from build123d import *

# Parameters (mm, degrees)
SKETCH1_W           = 56.4
SKETCH1_H           = 56.4
BOSS_EXTRUDE1_DEPTH = 56
SKETCH2_R           = 2.55
CUT_EXTRUDE1_DEPTH  = 6
SKETCH3_R           = 19.05
BOSS_EXTRUDE2_DEPTH = 1.6
SKETCH4_R           = 4
BOSS_EXTRUDE3_DEPTH = 23.9
FILLET1_R           = 4
SKETCH5_W           = 9.15
SKETCH5_H           = 9.15
CUT_EXTRUDE2_DEPTH  = 51
FILLET3_R           = 4
FILLET4_R           = 2


with BuildPart() as part:
    # Sketch1 → Boss-Extrude1 (new body)
    with BuildSketch(Plane.XY):
        Rectangle(SKETCH1_W, SKETCH1_H)
    extrude(amount=-BOSS_EXTRUDE1_DEPTH)

    # Sketch2 → Cut-Extrude1 (cut)
    with BuildSketch(Plane.XY):
        with Locations((-23.57, 23.57)):
            Circle(SKETCH2_R)
        with Locations((23.57, 23.57)):
            Circle(SKETCH2_R)
        with Locations((23.57, -23.57)):
            Circle(SKETCH2_R)
        with Locations((-23.57, -23.57)):
            Circle(SKETCH2_R)
    extrude(amount=-CUT_EXTRUDE1_DEPTH, mode=Mode.SUBTRACT)

    # Sketch3 → Boss-Extrude2 (add)
    with BuildSketch(Plane.XY):
        Circle(SKETCH3_R)
    extrude(amount=BOSS_EXTRUDE2_DEPTH)

    # Sketch4 → Boss-Extrude3 (add)
    with BuildSketch(Plane.XY.offset(1.6)):
        Circle(SKETCH4_R)
    extrude(amount=BOSS_EXTRUDE3_DEPTH)

    # Fillet1
    fillet1_edges = [part.edges().sort_by_distance(p)[0] for p in [
        (28.2, -28.2, -28),
        (-28.2, -28.2, -28),
        (-28.2, 28.2, -28),
        (28.2, 28.2, -28),
    ]]
    fillet(fillet1_edges, radius=FILLET1_R)

    # Sketch5 → Cut-Extrude2 (cut)
    with BuildSketch(Plane(origin=(0, 0, -56), x_dir=(-1, 0, 0), z_dir=(0, 0, -1))):
        with Locations((-23.625, 23.625)):
            Rectangle(SKETCH5_W, SKETCH5_H)
        with Locations((23.625, 23.625)):
            Rectangle(SKETCH5_W, SKETCH5_H)
        with Locations((23.625, -23.625)):
            Rectangle(SKETCH5_W, SKETCH5_H)
        with Locations((-23.625, -23.625)):
            Rectangle(SKETCH5_W, SKETCH5_H)
    extrude(amount=-CUT_EXTRUDE2_DEPTH, mode=Mode.SUBTRACT)

    # Fillet3
    fillet3_edges = [part.edges().sort_by_distance(p)[0] for p in [
        (-19.05, 19.05, -30.5),
        (19.05, 19.05, -30.5),
        (19.05, -19.05, -30.5),
        (-19.05, -19.05, -30.5),
    ]]
    fillet(fillet3_edges, radius=FILLET3_R)

    # Fillet4
    fillet4_edges = [part.edges().sort_by_distance(p)[0] for p in [
        (-28.2, 19.05, -30.5),
        (-19.05, 28.2, -30.5),
        (28.2, 19.05, -30.5),
        (19.05, 28.2, -30.5),
        (28.2, -19.05, -30.5),
        (19.05, -28.2, -30.5),
        (-28.2, -19.05, -30.5),
        (-19.05, -28.2, -30.5),
    ]]
    fillet(fillet4_edges, radius=FILLET4_R)


solid = part.part
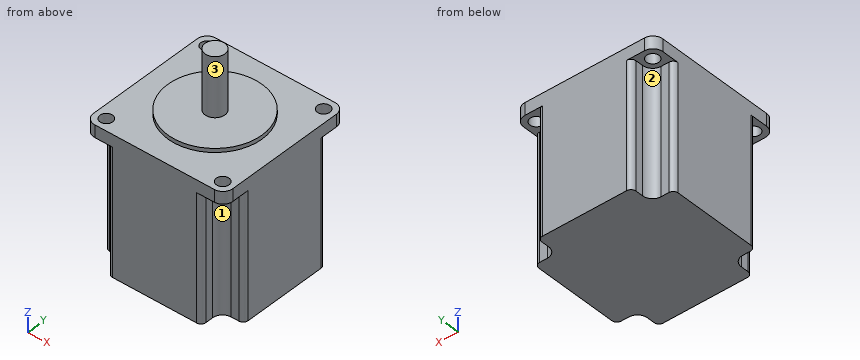
Geometry check sheet. Reference: the model listing, model coordinates, mm. Face numbers are marked on the shaded views. A direction names the side the tool comes from. Give positions to 0.01 mm unless a question says otherwise; leave off trailing zeros. Order: outer loops, then holes, each group sorted by start corner. A loop starts at its lowest first (then second) coordinate and runs counter-clockwise, first axis right, second up. Notation, with made-up numbers: (4.5, 35.5) - (29.5, 35.5) arc R19 ccw to (29.5, 51.5) - close; hole circle Ø10 at (-19, 21). An arc over 180 degrees is marked (long way). Answer as a JSON object with one key per item and string values.
(1) Material ranges on line 1 (Y direction, x = -23.57, z = -3); line 2 (X direction, y = -23, z = -1); line 3 (Y direction, x = 26.5, z = -12), recorded low to high.
Report:
{"line 1": "-28.2 to -26.12, -21.02 to 21.02, 26.12 to 28.2", "line 2": "-28.2 to -26.06, -21.08 to 21.08, 26.06 to 28.2", "line 3": "-19.03 to 19.03"}
(2) Tool access check on the marked faces 1, 2 and 3. Record the directions out of +Z, -Z, +X, -X, +Y, -Y that give a thin tool (end or side, any length) a straight path to the whole face; none if there is none.
Report:
{"face 1": "-Z, +X, -Y", "face 2": "-Z, -X, +Y", "face 3": "+Z"}
(3) Depth check by flat-ended pin: pin 1 Ø12.5 at (x, y) = (23, -24.5) entering from -Z; pin 2 Ø1.6 at (y, z) = (-25, -42.5) entering from -X; pin 3 Ø1.6 at (x, z) = (25, -22) entering from -Y; pin 4 Ø6 at (x, z) = (21, -35) entering from +Y. Enter the tip coordinate at first touch or a pass-through.
Report:
{"pin 1": "z = -56", "pin 2": "x = -19.05", "pin 3": "y = -19.05", "pin 4": "y = 27.96"}
(4) Cross-section at B-B (z = -20.5). Record the cut outline in (x, y).
Report:
{"outline": "(-28.2, -17.05) arc R2 ccw to (-26.2, -19.05) - (-23.05, -19.05) arc R4 cw to (-19.05, -23.05) - (-19.05, -26.2) arc R2 ccw to (-17.05, -28.2) - (17.05, -28.2) arc R2 ccw to (19.05, -26.2) - (19.05, -23.05) arc R4 cw to (23.05, -19.05) - (26.2, -19.05) arc R2 ccw to (28.2, -17.05) - (28.2, 17.05) arc R2 ccw to (26.2, 19.05) - (23.05, 19.05) arc R4 cw to (19.05, 23.05) - (19.05, 26.2) arc R2 ccw to (17.05, 28.2) - (-17.05, 28.2) arc R2 ccw to (-19.05, 26.2) - (-19.05, 23.05) arc R4 cw to (-23.05, 19.05) - (-26.2, 19.05) arc R2 ccw to (-28.2, 17.05) - close"}
(5) Cross-section at A-A (y = 0). Record the cut outline in (x, z).
Report:
{"outline": "(-28.2, -56) - (28.2, -56) - (28.2, 0) - (19.05, 0) - (19.05, 1.6) - (4, 1.6) - (4, 25.5) - (-4, 25.5) - (-4, 1.6) - (-19.05, 1.6) - (-19.05, 0) - (-28.2, 0) - close"}
(6) Cross-section at D-D (x = 10.5). Record the cut outline in (y, z).
Report:
{"outline": "(-28.2, -56) - (28.2, -56) - (28.2, 0) - (15.9, 0) - (15.9, 1.6) - (-15.9, 1.6) - (-15.9, 0) - (-28.2, 0) - close"}
